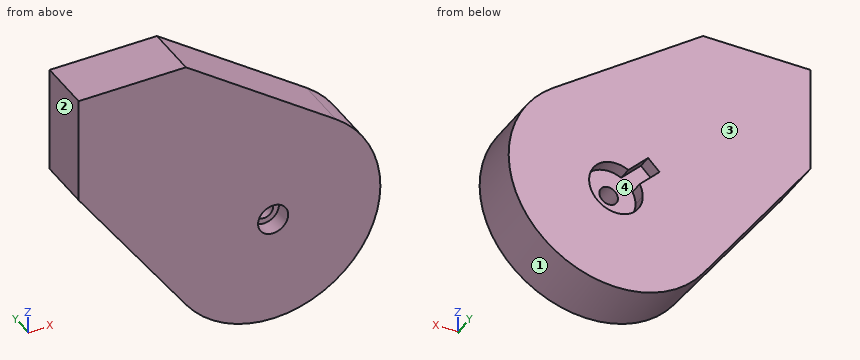
from build123d import *

# Parameters (mm, degrees)
F1_DEPTH       = 25.4
F3_D           = 8.8
F3_CBORE_D     = 14.25
F3_CBORE_DEPTH = 8
F5_DEPTH       = 6.35


with BuildPart() as f1:
    # F0 (on Front) → F1 (new body)
    with BuildSketch(Plane.XZ):
        with BuildLine():
            Line((-50.8, 50.8), (-50.8, 0))
            Line((-50.8, 0), (0, -70.8831193189))
            ThreePointArc((0, -70.8831193189), (77.2120156464, -77.2120156464), (70.8831193189, 0))
            Line((70.8831193189, 0), (0, 50.8))
            Line((0, 50.8), (-50.8, 50.8))
        make_face()
    extrude(amount=F1_DEPTH)

    # F3 (through all)
    with Locations(Plane.XZ.offset(25.4)):
        with Locations((41.2909911622, -41.2909911622)):
            CounterBoreHole(F3_D / 2, F3_CBORE_D / 2, F3_CBORE_DEPTH)

    # F4 (on face) → F5 (cut)
    with BuildSketch(Plane(origin=(0, 0, 0), x_dir=(-1, 0, 0), z_dir=(0, 1, 0))):
        with BuildLine():
            ThreePointArc((-35.4184496458, -30.0302959732), (-52.150808777, -47.8753940486), (-28.5909911622, -41.2909911622))
            ThreePointArc((-28.5909911622, -41.2909911622), (-28.9560645531, -38.2678164153), (-30.0302959732, -35.4184496458))
            Line((-30.0302959732, -35.4184496458), (-38.5969143258, -43.9850679985))
            Line((-38.5969143258, -43.9850679985), (-43.9850679985, -38.5969143258))
            Line((-43.9850679985, -38.5969143258), (-35.4184496458, -30.0302959732))
        make_face()
        with BuildLine():
            Line((-38.5969143258, -43.9850679985), (-30.0302959732, -35.4184496458))
            ThreePointArc((-30.0302959732, -35.4184496458), (-32.3107350411, -32.3107350411), (-35.4184496458, -30.0302959732))
            Line((-35.4184496458, -30.0302959732), (-43.9850679985, -38.5969143258))
            Line((-43.9850679985, -38.5969143258), (-38.5969143258, -43.9850679985))
        make_face()
        with BuildLine():
            ThreePointArc((-35.4184496458, -30.0302959732), (-32.3107350411, -32.3107350411), (-30.0302959732, -35.4184496458))
            Line((-30.0302959732, -35.4184496458), (-20.6364020837, -26.0245557563))
            Line((-20.6364020837, -26.0245557563), (-26.0245557563, -20.6364020837))
            Line((-26.0245557563, -20.6364020837), (-35.4184496458, -30.0302959732))
        make_face()
    extrude(amount=-F5_DEPTH, mode=Mode.SUBTRACT)


solid = f1.part
Design review of the part built by this model. Coordinates are the model's own, in mm. Face numbers are marked on the shaded views. Round coordinates to 2 decimals unless told otherwise and drop trailing zeros. Write each loop counter-clockwise with the first axis right and the second up, starting at its lowest first coordinate (ties: lowest second). Pieces come first, ordered by that corner, then holes. Notation, with made-up numbers: (77.5, 63) - (99.5, 63) arc R19 ccw to (99.5, 86) - close; hole circle Ø3 at (7, -36). An arc over 180 degrees is marked (long way). Return JSON: item names as keys, results as strings. Group by question number.
Item 1: The part is to be moulded in two halves that separate along X. For the marked faces 1, 2, 3 and 4, say which applies: pulls with the +X half, pulls with the -X half, needs draft (parallel to the pull), parting line crosses it, or undercut.
Item 2: We need section C-C on y = -22. Write out the cut boundary in (x, z) (3 decimals), and give its area (3 significant figures).
Item 3: We need section B-B on x = 44. Write out the cut boundary in (y, z), and give its area (3 significant figures).
Item 4: For probe 1 along X at (y, z) = (-4.25, -45.5); probe 2 along X at (y, z) = (-23, -39.5); probe 3 along Y at (x, z) = (39, -46.5), list the stretches that pass through material, from the lowest coordinate up. Write a range as [from, to].
Item 5: We need section D-D on z = 32.5. Write out the cut boundary in (x, y), and give its area (3 significant figures).
Item 6: We need section A-A on y = -3. Write out the cut boundary in (x, z), and give its area (3 significant figures).
Item 7: Insertion check: P1, Ø3, axis at x = 1.5, y = -14, coming from the -Z side; P2, Ø5, axis at y = -11, z = -32, coming from the -X side; P3, Ø5, axis at y = -13.5, z = 5.5, coming from the +X side. Each pin has a flat end and moves straight along its axis. Give the tip position at first contact, or say it passes through.
Model answer:
{
 "1": {"face 1": "parting line crosses it", "face 2": "pulls with the -X half", "face 3": "needs draft", "face 4": "undercut"},
 "2": {"outline": "(-50.8, 0) - (0, -70.883) arc R50.8 ccw (long way) to (70.883, 0) - (0, 50.8) - (-50.8, 50.8) - close; hole circle Ø14.25 at (41.291, -41.291)", "area": "13,400 mm²"},
 "3": {"outline": "(-25.4, -92.02) - (0, -92.02) - (0, -53.7) - (-6.35, -53.7) - (-6.35, -44.76) - (-17.4, -44.76) - (-17.4, -47.88) - (-25.4, -47.88) - close; (-25.4, -34.7) - (-17.4, -34.7) - (-17.4, -37.82) - (-6.35, -37.82) - (-6.35, -28.88) - (0, -28.88) - (0, 19.27) - (-25.4, 19.27) - close", "area": "2,490 mm²"},
 "4": {"probe 1": "x = [-18.19, 29.31], [53.27, 91.92]", "probe 2": "x = [-22.49, 34.39], [48.19, 92.06]", "probe 3": "y = [-17.4, -6.35]"},
 "5": {"outline": "(-50.8, -25.4) - (25.53, -25.4) - (25.53, 0) - (-50.8, 0) - close", "area": "1,940 mm²"},
 "6": {"outline": "(-50.8, 0) - (0, -70.88) arc R50.8 ccw (long way) to (70.88, 0) - (0, 50.8) - (-50.8, 50.8) - close; hole (20.64, -26.02) - (30.03, -35.42) arc R12.7 ccw (long way) to (35.42, -30.03) - (26.02, -20.64) - close", "area": "13,000 mm²"},
 "7": {"P1": "stops at z = -74.67", "P2": "stops at x = -29.66", "P3": "stops at x = 66.7"}
}
